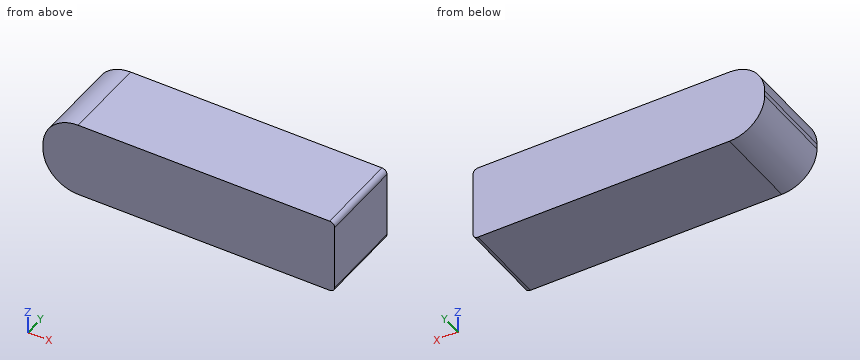
Autodesk Inventor part; units mm, degrees
ref_plane "YZ Plane" through (0, 0, 0) normal (1, 0, 0) x (0, 1, 0)
ref_plane "XZ Plane" through (0, 0, 0) normal (0, 1, 0) x (-1, 0, 0)
ref_plane "XY Plane" through (0, 0, 0) normal (0, 0, 1) x (1, 0, 0)
sketch "スケッチ1" plane through (0, 0, 0) normal (0, 0, 1) x (1, 0, 0)
  line L0 (-58, -17) -> (58, -17)
  line L1 (58, -17) -> (58, 17)
  line L2 (58, 17) -> (-58, 17)
  line L3 (-58, 17) -> (-58, -17)
  line L4 (-58, -17) -> (58, 17) construction
  line L5 (58, -17) -> (-58, 17) construction
  point P0 (0, 0)
  dimension "d0" = 116
  dimension "d1" = 34
extrude "押し出し1" add sketch "スケッチ1" along normal blind 15
mirror "ミラー1" about plane through (0, 0, 0) normal (0, 0, -1) of "押し出し1"
fillet "フィレット1" radius 14 2 edges at (-58, 0, 15) (-58, 0, -15)
fillet "フィレット2" radius 2 2 edges at (58, 0, 15) (58, 0, -15)
properties part number "HP-G570-2600S3"
Can you work these out from the model? Positions are in its coordinate system, mm. Give positions to 0.01 mm unless a question says otherwise; leave off trailing zeros. Write each loop counter-clockwise with the first axis right and the second up, starting at its lowest first coordinate (ties: lowest second). Pieces come first, ordered by that corner, then holes. Notation, with made-up numbers: (89, 43) -> (135, 43) arc R18 ccw to (135, 77) -> close; hole circle Ø3 at (49, -37.5). An arc over 180 degrees is marked (long way). Answer as a JSON object with one key per item and string values. Group by question number.
Item 1: Suppose I cut it at C-C (z = -10). Please give me the cut outline in (x, y).
Item 2: Suppose I cut it at B-B (z = 8). Please give me the cut outline in (x, y), plus the area to 3 significant figures.
Item 3: I'm going to push flat-ended pins straight in: P1, Ø1.5, axis at y = 5, z = 4.5, coming from the -X side; P2, Ø6, axis at y = -6, z = 5, coming from the -X side. Where does each tip first touch, or does it pass through?
Item 4: Please list where these lines run through material, in increasing order: line 1 (X direction, y = -4.5, z = 10.25); line 2 (X direction, y = -11, z = -9). Write a range as [from, to].
Item 5: Suppose I cut it at A-A (y = 9.5). Please give me the cut outline in (x, z), plus the area to 3 significant figures.
Findings:
{
 "1": {"outline": "(-54.72, -17) -> (58, -17) -> (58, 17) -> (-54.72, 17) -> close"},
 "2": {"outline": "(-56.12, -17) -> (58, -17) -> (58, 17) -> (-56.12, 17) -> close", "area": "3,880 mm²"},
 "3": {"P1": "stops at x = -57.73", "P2": "stops at x = -57.96"},
 "4": {"line 1": "x = [-54.51, 58]", "line 2": "x = [-55.49, 58]"},
 "5": {"outline": "(-58, -1) arc R14 ccw to (-44, -15) -> (56, -15) arc R2 ccw to (58, -13) -> (58, 13) arc R2 ccw to (56, 15) -> (-44, 15) arc R14 ccw to (-58, 1) -> close", "area": "3,390 mm²"}
}
